The model under review builds one solid part; all positions refer to its coordinate system, in mm. A direction names the side the tool comes from. Round coordinates to 2 decimals unless told otherwise and drop trailing zeros. Write each loop counter-clockwise with the first axis right and the second up, starting at its lowest first coordinate (ties: lowest second). Pieces come first, ordered by that corner, then holes. Notation, with made-up numbers: (-10.5, -28) -> (42.5, -28) arc R26 cw to (42.5, 7) -> close; hole circle Ø9 at (46.5, 48.25). An arc over 180 degrees is marked (long way). Answer in a Markdown table with one row per item. Add a question column.
```python
from build123d import *

# Parameters (mm, degrees)
F1_DEPTH = 127
F0_W     = 50.8
F0_H     = 50.8
F2_DEPTH = 127
F3_W     = 50.8
F3_H     = 50.8
F4_DEPTH = 76.2
F5_W     = 50.8
F5_H     = 50.8
F6_DEPTH = 76.2
F7_W     = 50.8
F7_H     = 50.8
F8_DEPTH = 101.6


with BuildPart() as f1:
    # F0 (on Front) → F1 (new body)
    with BuildSketch(Plane.XZ):
        Polygon((-29.016551, 16.690897), (-79.813677, 16.150502), (-79.813677, -34.109103), (-29.016551, -34.109103), align=None)
    extrude(amount=F1_DEPTH)

    # F3 (on face) → F4 (join)
    with BuildSketch(Plane(origin=(-0.180826, 0, 16.99766), x_dir=(0.999943, 0, 0.010638), z_dir=(-0.010638, 0, 0.999943))):
        with Locations((-54.237357, -25.4)):
            Rectangle(F3_W, F3_H)
    extrude(amount=F4_DEPTH)



with BuildPart() as f2:
    # F0 (on Front) → F2 (new body)
    with BuildSketch(Plane.XZ):
        with Locations((46.57851, -8.262248)):
            Rectangle(F0_W, F0_H)
    extrude(amount=F2_DEPTH)

    # F5 (on face) → F6 (join)
    with BuildSketch(Plane.XY.offset(17.137752)):
        with Locations((46.57851, -25.4)):
            Rectangle(F5_W, F5_H)
    extrude(amount=F6_DEPTH)


with BuildPart() as f1_1:
    add(f1.part)

    add(f2.part)  # F8 merges F2
    # F7 (on face) → F8 (join)
    with BuildSketch(Plane(origin=(-28.835725, 0, -0.306763), x_dir=(0, 1, 0), z_dir=(0.999943, 0, 0.010638))):
        with Locations((-25.4, 67.798622)):
            Rectangle(F7_W, F7_H)
    extrude(amount=F8_DEPTH)


solid = f1_1.part
```
1. Add section D-D on x = -44. Write out the cut boundary in (y, z), plus the area to 3 significant figures.
2. For L1, parallel to X at y = -112, z = -27; L2, parallel to Y at x = 5.5, z = 44.5; L3, parallel to Z at x = 25, y = -102, list the stretches that pass through material, from the lowest coordinate up.
3. Add section B-B on z = -12.5. Write out the cut boundary in (x, y), plus the area to 3 significant figures.
4. Insertion check: pin 1 Ø4 at (y, z) = (-70.5, 17) entering from +X; pin 2 Ø1 at (x, y) = (-6, -39.5) entering from +Z; pin 3 Ø5 at (x, y) = (29, -30.5) entering from -Z. Each pin has a flat end and moves straight along its axis. Give the tip position at first contact, or say it passes through.
5. Add section A-A on y = -99. Write out the cut boundary in (x, z), plus the area to 3 significant figures.
6. Mouldability with a two-part tool opening along X and no side actions: class faces 5 (the flat face through (71.979, -26, 84)), 6 (the flat face through (46, -127, -8)), 7 (the flat face through (-79.814, -63, -9)), 8 (the flat face through (21.179, -64, -5)) as pulls with the +X half, pulls with the -X half, needs draft (parallel to the pull), parting line crosses it, or undercut.
7. Tool access review of faces 1 (the flat face through (-5, 0, 45)), 2 (the flat face through (-29.017, -63, -9)), 3 (the flat face through (46, -88, 17.138)), 4 (the flat face through (46, -63, -33.662)): name each direction out of +Z, -Z, +X, -X, +Y, -Y from which nothing blocks a thin tool from reaching the whole face with its end or side.
Filled in:
| question | item | result |
|---|---|---|
| 1 | outline | (-127, -34.11) -> (0, -34.11) -> (0, 92.74) -> (-50.8, 92.74) -> (-50.8, 16.53) -> (-127, 16.53) -> close |
| 1 | area | 10,300 mm² |
| 2 | L1 | -79.81 to -29.02, 21.18 to 71.98 |
| 2 | L2 | -50.8 to 0 |
| 2 | L3 | -33.66 to 17.14 |
| 3 | outline | (-79.81, -127) -> (-29.02, -127) -> (-29.02, 0) -> (-79.81, 0) -> close; (21.18, -127) -> (71.98, -127) -> (71.98, 0) -> (21.18, 0) -> close |
| 3 | area | 12,900 mm² |
| 4 | pin 1 | x = 71.98 |
| 4 | pin 2 | z = 93.15 |
| 4 | pin 3 | z = -33.66 |
| 5 | outline | (-79.81, -34.11) -> (-29.02, -34.11) -> (-29.02, 16.69) -> (-79.81, 16.15) -> close; (21.18, -33.66) -> (71.98, -33.66) -> (71.98, 17.14) -> (21.18, 17.14) -> close |
| 5 | area | 5,150 mm² |
| 6 | face 5 | pulls with the +X half |
| 6 | face 6 | needs draft |
| 6 | face 7 | pulls with the -X half |
| 6 | face 8 | undercut |
| 7 | face 1 | +Z, -Z, +X, -X, +Y |
| 7 | face 2 | -Z, +Y, -Y |
| 7 | face 3 | +Z, +X, -X, -Y |
| 7 | face 4 | -Z, +X, +Y, -Y |
